from build123d import *

# Parameters (mm, degrees)
RESSALTO_EXTRUS_O1_DEPTH = 6
CORTE_EXTRUS_O1_DEPTH    = 3.1
ESBO_O4_R                = 15
CORTE_EXTRUS_O2_DEPTH    = 100.844211363
ESBO_O6_R                = 2
CORTE_EXTRUS_O3_DEPTH    = 3.1


with BuildPart() as part:
    # Esboço2 → Ressalto-extrusão1 (new body)
    with BuildSketch(Plane.XY):
        Polygon((70.472925804, 27.825776133), (30.15608873, 69.507678721), (-27.825776133, 70.472925804), (-69.507678721, 30.15608873), (-70.472925804, -27.825776133), (-30.15608873, -69.507678721), (27.825776133, -70.472925804), (69.507678721, -30.15608873), align=None)
    extrude(amount=RESSALTO_EXTRUS_O1_DEPTH)

    # Esboço3 → Corte-extrusão1 (cut)
    with BuildSketch(Plane.XY.offset(6)):
        Polygon((-61.0871998, -37.529288249), (-39.534791939, -59.811427182), (-25.159218434, -45.906647917), (-46.711626295, -23.624508984), align=None)
        Polygon((46.71864909, 23.617248408), (25.166241229, 45.899387341), (39.541814734, 59.804166606), (61.094222595, 37.522027673), align=None)
        Polygon((-59.804166606, 39.541814734), (-37.522027673, 61.094222595), (-23.617248408, 46.71864909), (-45.899387341, 25.166241229), align=None)
        Polygon((23.631531779, -46.718886871), (45.913670712, -25.16647901), (59.818449977, -39.542052515), (37.536311044, -61.094460376), align=None)
    extrude(amount=-CORTE_EXTRUS_O1_DEPTH, mode=Mode.SUBTRACT)

    # Esboço4 → Corte-extrusão2 (cut, through all)
    with BuildSketch(Plane.XY.offset(6)):
        Circle(ESBO_O4_R)
    extrude(amount=-CORTE_EXTRUS_O2_DEPTH, mode=Mode.SUBTRACT)

    # Esboço6 → Corte-extrusão3 (cut)
    with BuildSketch(Plane.XY.offset(2.9)):
        with Locations((-46.481705373, -31.053986514)):
            Circle(ESBO_O6_R)
        with Locations((-53.669492126, -38.006376147)):
            Circle(ESBO_O6_R)
        with Locations((-39.764712861, -52.381949652)):
            Circle(ESBO_O6_R)
        with Locations((-32.576926108, -45.429560019)):
            Circle(ESBO_O6_R)
        with Locations((39.779293109, 52.368949317)):
            Circle(ESBO_O6_R)
        with Locations((32.590503175, 45.417596982)):
            Circle(ESBO_O6_R)
        with Locations((53.681997779, 37.991369449)):
            Circle(ESBO_O6_R)
        with Locations((46.493207845, 31.040017114)):
            Circle(ESBO_O6_R)
        with Locations((38.006376147, -53.669492126)):
            Circle(ESBO_O6_R)
        with Locations((31.061009309, -46.488965949)):
            Circle(ESBO_O6_R)
        with Locations((52.381949652, -39.764712861)):
            Circle(ESBO_O6_R)
        with Locations((45.436582814, -32.584186684)):
            Circle(ESBO_O6_R)
        with Locations((-37.991369449, 53.681997779)):
            Circle(ESBO_O6_R)
        with Locations((-31.047038861, 46.500469435)):
            Circle(ESBO_O6_R)
        with Locations((-45.424618729, 32.597764765)):
            Circle(ESBO_O6_R)
        with Locations((-52.368949317, 39.779293109)):
            Circle(ESBO_O6_R)
    extrude(amount=-CORTE_EXTRUS_O3_DEPTH, mode=Mode.SUBTRACT)


solid = part.part
The model under review builds one solid part; all positions refer to its coordinate system, in mm. A direction names the side the tool comes from. Give positions to 0.01 mm unless a question says otherwise; leave off trailing zeros. Loops run counter-clockwise (first coordinate to the right, second up) from the corner with the lowest first, then second, coordinate; pieces in that order, holes last. Notation, with made-up numbers: (-33.5, -3.5) -> (-14.5, -3.5) arc R17 cw to (-14.5, 19.5) -> close; hole circle Ø5 at (39.5, 30). An arc over 180 degrees is marked (long way). Put each result on its own line as item: value. Start each with the question number.
1. We need section C-C on z = 4.7. State the section outline as (x, y) points.
2. Clearance check with flat-ended pins moving along their axes: P1, Ø4.5, axis at x = -53.67, y = -38.01, coming from the -Z side; P2, Ø3, axis at x = 45.44, y = -32.58, coming from the -Z side; P3, Ø1.5, axis at y = 50.5, z = 5.5, coming from the -X side; P4, Ø1, axis at x = 12.5, z = 5, coming from the -Y side. State where each tip first meets the part, or that it passes through.
3. For faces 4 (the face through (-30.67, -44.83, 1.47)), 5 (the face through (32.3, 52.8, 4.5)), 6 (the face through (-30.67, 54.01, 4.47)), 7 (the face through (-35.785, -34.922, 4.472)), list the 3-axis set-ups (+Z, -Z, +X, -X, +Y, -Y) from which the entire face can be reached by the end or side of a thin tool; tool diameter is ignored.
4. Wall thickness on probe 1 along Y at (x, z) = (-47, 2.75); probe 2 along X at (y, z) = (30, 5.6); probe 3 along Y at (x, z) = (-53.5, 4.8): over which ranges is each line inside the solid? List them lowest first.
5. We need section B-B on x = 3.5. State the section outline as (y, z) points, then the cut area to 3 significant figures.
6. We need section A-A on y = 0. State the section outline as (x, z) points.
7. Mouldability with a two-part tool opening along X and no side actions: class faces 1 (the face through (-1, 17, 6)), 2 (the face through (29.474, -47.706, 1.47)), 3 (the face through (50.6, 48.37, 2.29)) as released by +X, released by -X, zero draft, split by the parting line, or undercut.
Determined:
1. outline: (-70.47, -27.83) -> (-61.09, -37.53) -> (-46.71, -23.62) -> (-25.16, -45.91) -> (-39.53, -59.81) -> (-30.16, -69.51) -> (27.83, -70.47) -> (37.53, -61.09) -> (23.63, -46.72) -> (45.91, -25.17) -> (59.81, -39.53) -> (69.51, -30.16) -> (70.47, 27.83) -> (61.09, 37.52) -> (46.72, 23.62) -> (25.17, 45.9) -> (39.54, 59.8) -> (30.16, 69.51) -> (-27.83, 70.47) -> (-37.52, 61.09) -> (-23.62, 46.72) -> (-45.9, 25.17) -> (-59.8, 39.54) -> (-69.51, 30.16) -> close; hole circle Ø30 at (0, 0)
2. P1: z = 0
2. P2: through
2. P3: x = -28
2. P4: y = -70.23
3. face 4: +Z, -Z
3. face 5: +Z, +X
3. face 6: +Z, -X
3. face 7: +Z
4. probe 1: -52.09 to -32.99, -29.12 to 31.37, 33.83 to 51.93
4. probe 2: -69.51 to -50.57, -40.9 to 40.54, 53.32 to 68.37
4. probe 3: -30.19 to 33.02
5. outline: (-70.07, 0) -> (-14.59, 0) -> (-14.59, 6) -> (-70.07, 6) -> close; (14.59, 0) -> (69.95, 0) -> (69.95, 6) -> (14.59, 6) -> close
5. area: 665 mm^2
6. outline: (-70.01, 0) -> (-15, 0) -> (-15, 6) -> (-70.01, 6) -> close; (15, 0) -> (70.01, 0) -> (70.01, 6) -> (15, 6) -> close
7. face 1: zero draft
7. face 2: undercut
7. face 3: released by +X
